from build123d import *

# Parameters (mm, degrees)
F0_R     = 11
F1_DEPTH = 3.5


with BuildPart() as f1:
    # F0 (on Top) → F1 (new body, symmetric)
    with BuildSketch(Plane.XY):
        with BuildLine():
            ThreePointArc((4.8068902284, 23.1867481814), (3.40065434, 21.2355802686), (2.1143376362, 19.2033536732))
            ThreePointArc((2.1143376362, 19.2033536732), (1.0584202785, 19.2909091426), (0, 19.3396322429))
            ThreePointArc((0, 19.3396322429), (-1.0584202785, 19.2909091426), (-2.1143376362, 19.2033536732))
            ThreePointArc((-2.1143376362, 19.2033536732), (-3.40065434, 21.2355802686), (-4.8068902284, 23.1867481814))
            ThreePointArc((-4.8068902284, 23.1867481814), (-4.9615717482, 19.612078626), (-5.2325893193, 16.0443428904))
            ThreePointArc((-5.2325893193, 16.0443428904), (-13.3206225283, 7.9563096814), (-21.4086557373, 16.0443428904))
            ThreePointArc((-21.4086557373, 16.0443428904), (-20.3787118799, 19.4130691175), (-18.3847115054, 22.3170428173))
            ThreePointArc((-18.3847115054, 22.3170428173), (-31.1223848305, 17.5096597623), (-41.9289059937, 9.2284549028))
            ThreePointArc((-41.9289059937, 9.2284549028), (-45.5657635204, 0), (-41.9289059937, -9.2284549028))
            ThreePointArc((-41.9289059937, -9.2284549028), (-35.4148236465, -14.666894454), (-28.0357005491, -18.857173191))
            ThreePointArc((-28.0357005491, -18.857173191), (-30.3567973633, -14.31904571), (-30.0960739695, -9.2284549028))
            ThreePointArc((-30.0960739695, -9.2284549028), (-27.9226796708, -7.5682851491), (-25.1994561404, -7.3155798018))
            ThreePointArc((-25.1994561404, -7.3155798018), (-20.6333159795, -9.1010108427), (-17.0062072575, -12.399720028))
            ThreePointArc((-17.0062072575, -12.399720028), (-14.7799976822, -9.9240492174), (-11.9304154068, -8.2021793351))
            ThreePointArc((-11.9304154068, -8.2021793351), (-10.290534836, -8.2969879927), (-8.7665580213, -8.9099248871))
            ThreePointArc((-8.7665580213, -8.9099248871), (-3.6958082863, -14.3954527894), (0, -20.8873338997))
            ThreePointArc((0, -20.8873338997), (3.6958082863, -14.3954527894), (8.7665580213, -8.9099248871))
            ThreePointArc((8.7665580213, -8.9099248871), (10.290534836, -8.2969879927), (11.9304154068, -8.2021793351))
            ThreePointArc((11.9304154068, -8.2021793351), (14.7799976822, -9.9240492174), (17.0062072575, -12.399720028))
            ThreePointArc((17.0062072575, -12.399720028), (20.6333159795, -9.1010108427), (25.1994561404, -7.3155798018))
            ThreePointArc((25.1994561404, -7.3155798018), (27.9226796708, -7.5682851491), (30.0960739695, -9.2284549028))
            ThreePointArc((30.0960739695, -9.2284549028), (30.3567973633, -14.31904571), (28.0357005491, -18.857173191))
            ThreePointArc((28.0357005491, -18.857173191), (35.4148236465, -14.666894454), (41.9289059937, -9.2284549028))
            ThreePointArc((41.9289059937, -9.2284549028), (45.5657635204, 0), (41.9289059937, 9.2284549028))
            ThreePointArc((41.9289059937, 9.2284549028), (31.1223848305, 17.5096597623), (18.3847115054, 22.3170428173))
            ThreePointArc((18.3847115054, 22.3170428173), (20.3787118799, 19.4130691175), (21.4086557373, 16.0443428904))
            ThreePointArc((21.4086557373, 16.0443428904), (13.3206225283, 7.9563096814), (5.2325893193, 16.0443428904))
            ThreePointArc((5.2325893193, 16.0443428904), (4.9615717482, 19.612078626), (4.8068902284, 23.1867481814))
        make_face()
        Circle(F0_R, mode=Mode.SUBTRACT)
    extrude(amount=F1_DEPTH, both=True)


solid = f1.part
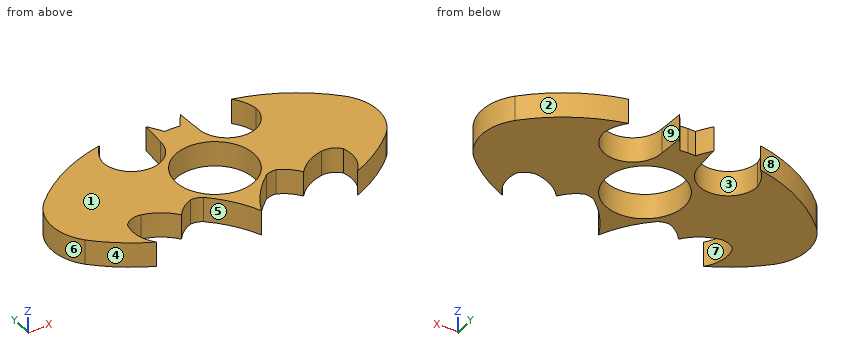
The model under review builds one solid part; all positions refer to its coordinate system, in mm. Face numbers are marked on the shaded views. A direction names the side the tool comes from. Round coordinates to 2 decimals unless told otherwise and drop trailing zeros. Write each loop counter-clockwise with the first axis right and the second up, starting at its lowest first coordinate (ties: lowest second). Pieces come first, ordered by that corner, then holes. Notation, with made-up numbers: M -11,-32.75 L 32,-32.75 A30 cw 32,-2.75 Z; hole C -2.75,-20.5 d11. An arc over 180 degrees is marked long. Use a Markdown table: item, result. Add a question column.
Q1. We need section B-B, the plane y = 0. State the section outline as (x, z) points, plus the area to 3 significant figures.
Q2. To check wall thickness, follow line 1 (X direction, y = 17, z = 2.25); line 2 (X direction, y = 13, z = -2); line 3 (Y direction, x = 19.5, z = 1.5). State the ranges of each line that lie inside material, in increasing order.
Q3. The part is to be moulded in two halves that separate along X. For the marked faces 1, 2, 3 and 4, say which applies: pulls with the +X half, pulls with the -X half, needs draft (parallel to the pull), parting line crosses it, or undercut.
Q4. We need section D-D, the plane x = 40. State the section outline as (y, z) points, plus the area to 3 significant figures.
Q5. Machinability: for the marked faces 5, 6, 7, 8 and 9, which of the approach directions +Z, -Z, +X, -X, +Y, -Y give a long, thin tool a straight path to every point of the face, cutting with its end or side? Answer none if there is none.
Q6. We need section C-C, the plane y = 14.5. State the section outline as (x, z) points, plus the area to 3 significant figures.
Q7. Insertion check: pin 1 (4 mm diameter, centred on x = 18, z = 1, fed in from -Y); pin 2 (1.5 mm diameter, centred on x = 11, z = 2, fed in from +Y). Each pin has a flat end and moves straight along its axis. Give the tip position at first contact, or say it passes through.
Findings below:
| question | item | result |
|---|---|---|
| 1 | outline | M -45.57,-3.5 L -11,-3.5 L -11,3.5 L -45.57,3.5 Z; M 11,-3.5 L 45.57,-3.5 L 45.57,3.5 L 11,3.5 Z |
| 1 | area | 484 mm² |
| 2 | line 1 | x = -32.02 to -21.23, -5.15 to 5.15, 21.23 to 32.02 |
| 2 | line 2 | x = -37.8 to -20.81, -5.83 to 5.83, 20.81 to 37.8 |
| 2 | line 3 | y = -9.89 to 10.83, 20.93 to 22.06 |
| 3 | face 1 | needs draft |
| 3 | face 2 | pulls with the +X half |
| 3 | face 3 | undercut |
| 3 | face 4 | pulls with the -X half |
| 4 | outline | M -11.05,-3.5 L 11.1,-3.5 L 11.1,3.5 L -11.05,3.5 Z |
| 4 | area | 155 mm² |
| 5 | face 5 | +Z, -Z, -Y |
| 5 | face 6 | +Z, -Z, -X |
| 5 | face 7 | +Z, -Z |
| 5 | face 8 | +Z, -Z, -X, +Y |
| 5 | face 9 | +Z, -Z, +Y |
| 6 | outline | M -35.84,-3.5 L -21.26,-3.5 L -21.26,3.5 L -35.84,3.5 Z; M -5.38,-3.5 L 5.38,-3.5 L 5.38,3.5 L -5.38,3.5 Z; M 21.26,-3.5 L 35.84,-3.5 L 35.84,3.5 L 21.26,3.5 Z |
| 6 | area | 280 mm² |
| 7 | pin 1 | stops at y = -12.4 |
| 7 | pin 2 | stops at y = 8.56 |
